Model file for the job. Use its own axes, mm. Face numbers are marked on the shaded views. A direction names the side the tool comes from. Give positions to 0.01 mm unless a question says otherwise; leave off trailing zeros. Write each loop counter-clockwise with the first axis right and the second up, starting at its lowest first coordinate (ties: lowest second). Pieces come first, ordered by that corner, then holes. Notation, with made-up numbers: (-37.75, 20.5) - (5.25, 20.5) arc R30 ccw to (5.25, 53.5) - close; hole circle Ø4 at (35, 47). An arc over 180 degrees is marked (long way). One line per item, written item: value. Start each with the question number.
(1) Cut at C-C, the plane x = 3.5. List the corners of the cut face in (y, z), and give its area (3 significant figures).
(2) Drop a flat-ended pin along its axis: P1, Ø2, axis at x = 2.5, z = 4.5, coming from the +Y side. Give the stop position or say it passes through.
(3) Mould opens along X. For the marked faces 4, 5, 6 and 7 say: pulls with the +X half, pulls with the -X half, needs draft (parallel to the pull), parting line crosses it, or undercut.
(4) 3-axis set-ups, long thin cutter, end or side, ignore diameter. For the marked faces 1, 2 and 3: which of +Z, -Z, +X, -X, +Y, -Y reach the whole face in a straight line?
(5) Probe L1, parallel to X at y = -17, z = 2.3; L2, parallel to Y at x = -3.75, z = 2.1; L3, parallel to Y at x = 4, z = 0.6. List the from-to ranges inside material, lowest first.
(6) Cut at A-A, the plane y = -19.5. List the corners of the cut face in (x, z), and give its area (3 significant figures).
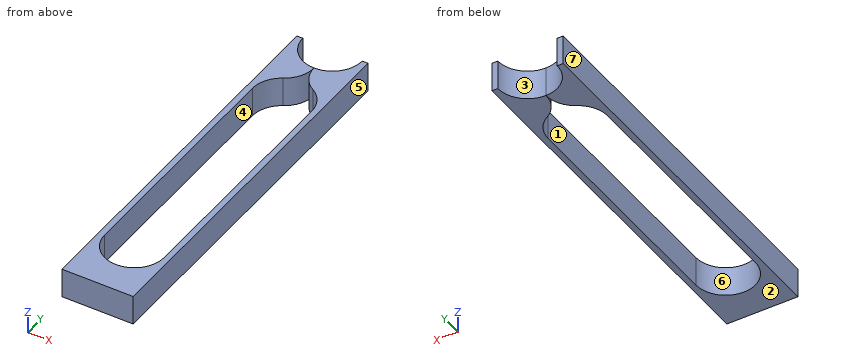
from build123d import *

# Parameters (mm, degrees)
PAD_DEPTH = 5


with BuildPart() as part:
    # Sketch → Pad (new body)
    with BuildSketch(Plane.XY):
        with BuildLine():
            ThreePointArc((-5, 13.660254), (-3.535534, 10.12472), (0, 8.660254))
            ThreePointArc((-2.5, 4.330127), (-0.669873, 6.160254), (0, 8.660254))
            ThreePointArc((-2.5, 4.330127), (-4.330127, 2.5), (-5, 0))
            Line((-5, 0), (-5, -40))
            ThreePointArc((-5, -40), (0, -45), (5, -40))
            Line((5, -40), (5, 0))
            ThreePointArc((5, 0), (4.330127, 2.5), (2.5, 4.330127))
            ThreePointArc((0, 8.660254), (0.669873, 6.160254), (2.5, 4.330127))
            ThreePointArc((0, 8.660254), (3.535534, 10.12472), (5, 13.660254))
            Line((5, 13.660254), (6, 13.660254))
            Line((6, 13.660254), (6, -50))
            Line((6, -50), (-6, -50))
            Line((-6, -50), (-6, 13.660254))
            Line((-6, 13.660254), (-5, 13.660254))
        make_face()
    extrude(amount=PAD_DEPTH)


solid = part.part
Answers follow:
1. outline: (-50, 0) - (-43.57, 0) - (-43.57, 5) - (-50, 5) - close; (3.57, 0) - (10.09, 0) - (10.09, 5) - (3.57, 5) - close
1. area: 64.7 mm²
2. P1: stops at y = 10.09
3. face 4: undercut
3. face 5: pulls with the +X half
3. face 6: undercut
3. face 7: pulls with the -X half
4. face 1: +Z, -Z
4. face 2: -Z, +X, -X, +Y, -Y
4. face 3: +Z, -Z, +Y
5. L1: x = -6 to -5, 5 to 6
5. L2: y = -50 to -43.31, 3.31 to 10.35
5. L3: y = -50 to -43, 3 to 10.66
6. outline: (-6, 0) - (-5, 0) - (-5, 5) - (-6, 5) - close; (5, 0) - (6, 0) - (6, 5) - (5, 5) - close
6. area: 10.0 mm²
